```python
from build123d import *

# Parameters (mm, degrees)
F1_DEPTH = 2
F4_COUNT = 6
F4_ANGLE = 300


with BuildPart() as f1:
    # F0 (on Top) → F1 (new body)
    with BuildSketch(Plane.XY):
        with BuildLine():
            Line((0, 95), (0, 82.2314136744))
            ThreePointArc((0, 82.2314136744), (1.6812792043, 81.736834508), (3.4327861377, 81.677405755))
            ThreePointArc((3.4327861377, 81.677405755), (9.5389305529, 90.3543086779), (0, 95))
        make_face()
        with BuildLine():
            ThreePointArc((3.4327861377, 81.677405755), (1.6812792043, 81.736834508), (0, 82.2314136744))
            Line((0, 82.2314136744), (0, 0))
            Line((0, 0), (5.8111646213, 0))
            Line((5.8111646213, 0), (32.2307050228, 51.1501394212))
            Line((32.2307050228, 51.1501394212), (30.095031485, 62.3711198568))
            Line((30.095031485, 62.3711198568), (6.0886708088, 29.0896948427))
            Line((6.0886708088, 29.0896948427), (5.0296979025, 40.3754748404))
            Line((5.0296979025, 40.3754748404), (20.4256810248, 68.0427178741))
            Line((20.4256810248, 68.0427178741), (2.5684384163, 66.1806464195))
            Line((2.5684384163, 66.1806464195), (21.2782546878, 80.7941183448))
            Line((21.2782546878, 80.7941183448), (3.4327861377, 81.677405755))
        make_face()
    extrude(amount=F1_DEPTH)

    # F2: F1 across plane


with BuildPart() as f1_1:
    add(f1.part)
    add(f1.part.mirror(Plane.YZ))

    # F4: F1 ×6 about axis
    f4_axis = Axis((0, 0, 4.1130185127), (0, 0, 1))


with BuildPart() as f1_2:
    add(f1_1.part)
    for i in range(1, F4_COUNT):
        add(f1_1.part.rotate(f4_axis, i * F4_ANGLE / (F4_COUNT - 1)))


solid = f1_2.part
```
For this review, take the finished solid that the model builds, in its own axes (mm). Coordinates: 2 decimals unless noted, no trailing zeros. Write each loop counter-clockwise with the first axis right and the second up, starting at its lowest first coordinate (ties: lowest second). Pieces come first, ordered by that corner, then holes. Notation, with made-up numbers: (-10, 59.5) - (45, 59.5) arc R25 cw to (45, 91.5) - close; hole circle Ø4 at (14, -13). An arc over 180 degrees is marked (long way). Answer in a Markdown table with one row per item. Add a question column.
Q1. We need section A-A, the plane x = -51.5. State the section outline as (y, z) points.
Q2. For P1, Ø1, axis at x = 22, z = 0.5, coming from the -Y side, flat-tipped, find the tip position at first contact; note if it passes through.
Q3. For probe 1 along X at (y, z) = (33, 1.4); probe 2 along X at (y, z) = (-21, 1.75); probe 3 along Y at (x, z) = (23.5, 0.65), list the stretches that pass through material, from the lowest coordinate up.
Q4. We need section B-B, the plane y = -74.5. State the section outline as (x, z) points, and give its area (3 significant figures).
Q5. We need section C-C, the plane y = 11.5. State the section outline as (x, z) points, and give its area (3 significant figures).
Q6. Draft analysis for pull direction X (two halves, no side actions). For faces 1 (the flat face through (66.051, -2.525, 0.986)), 2 (the flat face through (69.4, -26.5, 1)), state which applies: +X half, -X half, draft (parallel to the pull), parting line (faces both ways), or undercut.
Answer list:
| question | item | result |
|---|---|---|
| 1 | outline | (-45.47, 0) - (-16.05, 0) - (-16.05, 2) - (-45.47, 2) - close; (-6.91, 0) - (6.91, 0) - (6.91, 2) - (-6.91, 2) - close; (16.05, 0) - (45.47, 0) - (45.47, 2) - (16.05, 2) - close |
| 2 | P1 | stops at y = -51.84 |
| 3 | probe 1 | x = -74.95 to -37.51, -28.07 to -8.91, -5.72 to 5.72, 8.91 to 28.07, 37.51 to 74.95 |
| 3 | probe 2 | x = -65.75 to -24.73, -22.68 to 22.68, 24.73 to 65.75 |
| 3 | probe 3 | y = -53.23 to -22.83, -20.44 to 20.44, 22.83 to 53.23 |
| 4 | outline | (-13.22, 0) - (13.22, 0) - (13.22, 2) - (-13.22, 2) - close |
| 4 | area | 52.9 mm2 |
| 5 | outline | (-31.38, 0) - (31.38, 0) - (31.38, 2) - (-31.38, 2) - close |
| 5 | area | 126 mm2 |
| 6 | face 1 | +X half |
| 6 | face 2 | undercut |
